Can you work these out from the model? Positions are in its coordinate system, mm. A direction names the side the tool comes from. Give positions to 0.01 mm unless a question says otherwise; leave off trailing zeros. Order: outer loops, then holes, each group sorted by start corner. A loop starts at its lowest first (then second) coordinate and runs counter-clockwise, first axis right, second up. Notation, with made-up numbers: (53.25, 8) - (81.25, 8) arc R24 cw to (81.25, 37) - close; hole circle Ø10 at (52.5, 78). An arc over 180 degrees is marked (long way). Answer as a JSON object with one key per item and string values.
```python
from build123d import *

# Parameters (mm, degrees)
BOSS_EXTRUDE1_DEPTH = 3.175
SKETCH2_R           = 3.4925
CUT_EXTRUDE2_DEPTH  = 3.175
LPATTERN5_COUNT     = 2
LPATTERN5_PITCH     = 22.86
SKETCH7_R           = 3.4925
CUT_EXTRUDE3_DEPTH  = 3.175
LPATTERN6_COUNT     = 3
LPATTERN6_PITCH     = 22.86
SKETCH8_R           = 3.4925
CUT_EXTRUDE4_DEPTH  = 62.882370874
FILLET1_R           = 12.7
FILLET2_R           = 3.175


with BuildPart() as part:
    # Sketch1 → Boss-Extrude1 (new body)
    with BuildSketch(Plane(origin=(0, 0, 0), x_dir=(1, 0, 0), z_dir=(0, 1, 0))):
        Polygon((-17.960512242, 17.960512242), (0, 35.921024484), (17.960512242, 17.960512242), (50.289434278, -14.368409794), (32.328922036, -32.328922036), (0, 0), (-32.328922036, -32.328922036), (-50.289434278, -14.368409794), align=None)
    extrude(amount=BOSS_EXTRUDE1_DEPTH)

    # Sketch2 → Cut-Extrude2 (cut)
    with BuildSketch(Plane(origin=(0, 3.175, 0), x_dir=(1, 0, 0), z_dir=(0, 1, 0))):
        with Locations(Location((-33.226947648, -15.266435406, 0), (0, 0, 270))):
            Circle(SKETCH2_R)
    cut_extrude2 = extrude(amount=-CUT_EXTRUDE2_DEPTH, mode=Mode.SUBTRACT)

    # LPattern5: Cut-Extrude2 ×2
    with Locations(*[Vector(0.7071067811865465, 0, -0.7071067811865487) * (i * LPATTERN5_PITCH) for i in range(1, LPATTERN5_COUNT)]):
        add(cut_extrude2, mode=Mode.SUBTRACT)

    # Sketch7 → Cut-Extrude3 (cut)
    with BuildSketch(Plane(origin=(0, 3.175, 0), x_dir=(1, 0, 0), z_dir=(0, 1, 0))):
        with Locations(Location((33.226947648, -15.266435406, 0), (0, 0, 270))):
            Circle(SKETCH7_R)
    cut_extrude3 = extrude(amount=-CUT_EXTRUDE3_DEPTH, mode=Mode.SUBTRACT)

    # LPattern6: Cut-Extrude3 ×3
    with Locations(*[Vector(-0.7071067811865456, 0, -0.7071067811865496) * (i * LPATTERN6_PITCH) for i in range(1, LPATTERN6_COUNT)]):
        add(cut_extrude3, mode=Mode.SUBTRACT)

    # Sketch8 → Cut-Extrude4 (cut, through all)
    with BuildSketch(Plane(origin=(0, 3.175, 0), x_dir=(1, 0, 0), z_dir=(0, 1, 0))):
        Polygon((16.164461018, -16.164461018), (32.328922036, -32.328922036), (50.289434278, -14.368409794), (34.12497326, 1.796051224), align=None)
        with Locations((33.226947648, -15.266435406)):
            Circle(SKETCH8_R, mode=Mode.SUBTRACT)
    extrude(amount=-CUT_EXTRUDE4_DEPTH, mode=Mode.SUBTRACT)

    # Fillet1
    fillet1_edges = [part.edges().sort_by_distance(p)[0] for p in [
        (0, 1.5875, 0),
    ]]
    fillet(fillet1_edges, radius=FILLET1_R)

    # Fillet2
    fillet2_edges = [part.edges().sort_by_distance(p)[0] for p in [
        (0, 1.5875, -35.921024484),
        (-32.328922036, 1.5875, 32.328922036),
        (-50.289434278, 1.5875, 14.368409794),
        (16.164461018, 1.5875, 16.164461018),
        (34.12497326, 1.5875, -1.796051224),
    ]]
    fillet(fillet2_edges, radius=FILLET2_R)


solid = part.part
```
Q1. If we section it at B-B, the plane z = -15.5: Please give me the cut outline in (x, y) (3 decimals).
Recorded:
{"outline": "(-20.421, 0) - (-2.225, 0) - (-2.225, 3.175) - (-20.421, 3.175) - close; (4.022, 0) - (20.421, 0) - (20.421, 3.175) - (4.022, 3.175) - close"}
Q2. Which directions (+Z, -Z, +X, -X, +Y, -Y) give clear straight access to the entire face, cutting with the end or side of a thin tool? Please do faces 5 (the face through (11, 2, 11)), 6 (the face through (25.24, 1.61, 7.09)).
Recorded:
{"face 5": "+Z, +Y, -Y", "face 6": "+Z, +X, +Y, -Y"}
Q3. We'd pull the mould along Z, two halves only. Please class faces 1 (the face through (-36.325, 1.61, 16.878)), 2 (the face through (-0.44, 1.61, -13.836)), 3 (the face through (-48.974, 1.61, 14.403)), 4 (the face through (-8, 3.175, -2)): released by +Z, released by -Z, zero draft, split by the parting line, or undercut.
Recorded:
{"face 1": "undercut", "face 2": "undercut", "face 3": "split by the parting line", "face 4": "zero draft"}
Q4. If we section it at D-D, the plane x = 22: Please give me the cut outline in (y, z) (3 decimals), then the cut area to 3 significant figures.
Recorded:
{"outline": "(0, -13.921) - (3.175, -13.921) - (3.175, 10.329) - (0, 10.329) - close", "area": "77.0 mm^2"}
Q5. I need wall thicknesses on L1, parallel to X at y = 0.85, z = -1.5; L2, parallel to Z at x = 3.5, y = 0.35; L3, parallel to X at y = 1.65, z = -18. Which ranges of each line are inside material? Lowest first, please.
Recorded:
{"L1": "x = -34.42 to -20.5, -13.62 to 13.62, 20.5 to 32.8", "L2": "z = -32.42 to -19.39, -14.73 to 5.75", "L3": "x = -17.92 to -2.47, 4.26 to 17.92"}
Q6. I'm going to push a flat-ended pin straight in: pin 1 Ø5 at (x, z) = (11, -26.5) entering from +Y (3 decimals). Where does the tip first touch, or does it pass through?
Recorded:
{"pin 1": "stops at y = 3.175"}
Q7. If we section it at A-A, the plane y = 2.35: Count the separate pieces of the cut face and the enclosed holes in it, then the cut area to 3 significant figures.
Recorded:
{"separate pieces": "1", "enclosed holes": "4", "area": "2,260 mm^2"}
Q8. If we section it at C-C, the plane x = -15.5: Please give me the cut outline in (y, z) (3 decimals), then the cut area to 3 significant figures.
Recorded:
{"outline": "(0, -20.421) - (3.175, -20.421) - (3.175, -4.022) - (0, -4.022) - close; (0, 2.225) - (3.175, 2.225) - (3.175, 15.5) - (0, 15.5) - close", "area": "94.2 mm^2"}
